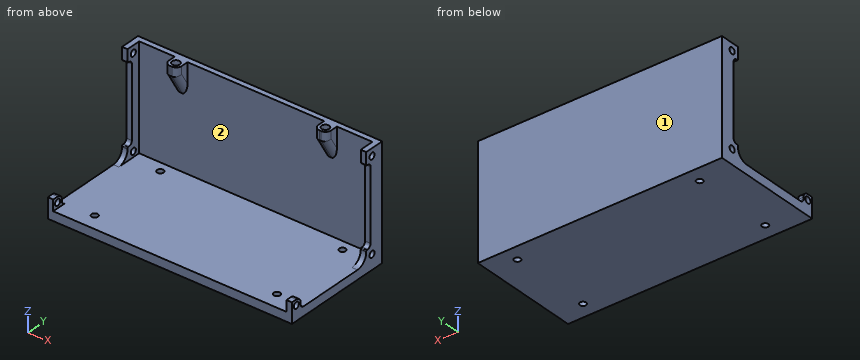
from build123d import *

# Parameters (mm, degrees)
SKETCH_W        = 134
SKETCH_H        = 62
PAD_DEPTH       = 5
SKETCH001_W     = 134
SKETCH001_H     = 3
PAD001_DEPTH    = 57
SKETCH002_W     = 7
SKETCH002_H     = 17
PAD002_DEPTH    = 7
POCKET_DEPTH    = 89
FILLET_R        = 3
SKETCH004_W     = 3
SKETCH004_H     = 57
PAD003_DEPTH    = 5
SKETCH005_W     = 3
SKETCH005_H     = 7
PAD004_DEPTH    = 3
SKETCH006_R     = 1.75
POCKET001_DEPTH = 134.001
SKETCH007_R     = 1.75
POCKET002_DEPTH = 5
SKETCH008_R     = 1.75
POCKET003_DEPTH = 5
SKETCH009_W     = 3
SKETCH009_H     = 6
PAD005_DEPTH    = 6
SKETCH010_R     = 1.75
POCKET004_DEPTH = 134.001
FILLET001_R     = 3
FILLET002_R     = 2
FILLET003_R     = 3
FILLET004_R     = 2
FILLET005_R     = 6
FILLET006_R     = 6
FILLET007_R     = 2
FILLET008_R     = 0.5
FILLET009_R     = 2
FILLET010_R     = 0.5
FILLET011_R     = 2
FILLET012_R     = 0.5
FILLET013_R     = 2
FILLET014_R     = 0.5
SKETCH011_R     = 1.75
POCKET005_DEPTH = 5
SKETCH012_R     = 2.1
POCKET006_DEPTH = 5


with BuildPart() as part:
    # Sketch → Pad (new body)
    with BuildSketch(Plane.XY):
        with Locations((67, -31)):
            Rectangle(SKETCH_W, SKETCH_H)
    extrude(amount=PAD_DEPTH)

    # Sketch001 (on Face6 of Pad) → Pad001 (join)
    with BuildSketch(Plane.XY.offset(5)):
        with Locations((67, -1.5)):
            Rectangle(SKETCH001_W, SKETCH001_H)
    extrude(amount=PAD001_DEPTH)

    # Sketch002 (on Face11 of Pad001) → Pad002 (join)
    with BuildSketch(Plane.XZ.offset(3)):
        with Locations((26, 53.5)):
            Rectangle(SKETCH002_W, SKETCH002_H)
        with Locations((108, 53.5)):
            Rectangle(SKETCH002_W, SKETCH002_H)
    extrude(amount=PAD002_DEPTH)

    # Sketch003 (on Face14 of Pad002) → Pocket (cut)
    with BuildSketch(Plane(origin=(22.5, 0, 0), x_dir=(0, -1, 0), z_dir=(-1, 0, 0))):
        Polygon((3, 45), (10, 57), (10, 45), align=None)
    extrude(amount=-POCKET_DEPTH, mode=Mode.SUBTRACT)

    # Fillet
    fillet_edges = [part.edges().sort_by_distance(p)[0] for p in [
        (104.5, -10, 59.5),
        (111.5, -10, 59.5),
        (111.5, -6.5, 51),
        (104.5, -6.5, 51),
        (22.5, -10, 59.5),
        (29.5, -10, 59.5),
        (29.5, -6.5, 51),
        (22.5, -6.5, 51),
    ]]
    fillet(fillet_edges, radius=FILLET_R)

    # Sketch004 (on Face1 of Fillet) → Pad003 (join)
    with BuildSketch(Plane.XZ.offset(3)):
        with Locations((1.5, 33.5)):
            Rectangle(SKETCH004_W, SKETCH004_H)
        with Locations((132.5, 33.5)):
            Rectangle(SKETCH004_W, SKETCH004_H)
    extrude(amount=PAD003_DEPTH)

    # Sketch005 (on Face32 of Pad003) → Pad004 (join)
    with BuildSketch(Plane.XZ.offset(8)):
        with Locations((1.5, 8.5)):
            Rectangle(SKETCH005_W, SKETCH005_H)
        with Locations((1.5, 58.5)):
            Rectangle(SKETCH005_W, SKETCH005_H)
        with Locations((132.5, 8.5)):
            Rectangle(SKETCH005_W, SKETCH005_H)
        with Locations((132.5, 58.5)):
            Rectangle(SKETCH005_W, SKETCH005_H)
    extrude(amount=PAD004_DEPTH)

    # Sketch006 (on Face44 of Pad004) → Pocket001 (cut, through all)
    with BuildSketch(Plane(origin=(0, 0, 0), x_dir=(0, -1, 0), z_dir=(-1, 0, 0))):
        with Locations((7, 8)):
            Circle(SKETCH006_R)
    extrude(amount=-POCKET001_DEPTH, mode=Mode.SUBTRACT)

    # Sketch007 (on Face46 of Pocket001) → Pocket002 (cut)
    with BuildSketch(Plane(origin=(0, 0, 0), x_dir=(0, -1, 0), z_dir=(-1, 0, 0))):
        with Locations((7, 58)):
            Circle(SKETCH007_R)
    extrude(amount=-POCKET002_DEPTH, mode=Mode.SUBTRACT)

    # Sketch008 (on Face45 of Pocket002) → Pocket003 (cut)
    with BuildSketch(Plane.YZ.offset(134)):
        with Locations((-7, 58)):
            Circle(SKETCH008_R)
    extrude(amount=-POCKET003_DEPTH, mode=Mode.SUBTRACT)

    # Sketch009 (on Face10 of Pocket003) → Pad005 (join)
    with BuildSketch(Plane.XY.offset(5)):
        with Locations((1.5, -59)):
            Rectangle(SKETCH009_W, SKETCH009_H)
        with Locations((132.5, -59)):
            Rectangle(SKETCH009_W, SKETCH009_H)
    extrude(amount=PAD005_DEPTH)

    # Sketch010 (on Face60 of Pad005) → Pocket004 (cut, through all)
    with BuildSketch(Plane.YZ.offset(134)):
        with Locations((-59, 8)):
            Circle(SKETCH010_R)
    extrude(amount=-POCKET004_DEPTH, mode=Mode.SUBTRACT)

    # Fillet001
    fillet001_edges = [part.edges().sort_by_distance(p)[0] for p in [
        (132.5, -56, 11),
    ]]
    fillet(fillet001_edges, radius=FILLET001_R)

    # Fillet002
    fillet002_edges = [part.edges().sort_by_distance(p)[0] for p in [
        (132.5, -56, 5),
    ]]
    fillet(fillet002_edges, radius=FILLET002_R)

    # Fillet003
    fillet003_edges = [part.edges().sort_by_distance(p)[0] for p in [
        (1.5, -56, 11),
    ]]
    fillet(fillet003_edges, radius=FILLET003_R)

    # Fillet004
    fillet004_edges = [part.edges().sort_by_distance(p)[0] for p in [
        (1.5, -56, 5),
    ]]
    fillet(fillet004_edges, radius=FILLET004_R)

    # Fillet005
    fillet005_edges = [part.edges().sort_by_distance(p)[0] for p in [
        (1.5, -11, 5),
    ]]
    fillet(fillet005_edges, radius=FILLET005_R)

    # Fillet006
    fillet006_edges = [part.edges().sort_by_distance(p)[0] for p in [
        (132.5, -11, 5),
    ]]
    fillet(fillet006_edges, radius=FILLET006_R)

    # Fillet007
    fillet007_edges = [part.edges().sort_by_distance(p)[0] for p in [
        (1.5, -8, 12),
    ]]
    fillet(fillet007_edges, radius=FILLET007_R)

    # Fillet008
    fillet008_edges = [part.edges().sort_by_distance(p)[0] for p in [
        (1.5, -11, 12),
    ]]
    fillet(fillet008_edges, radius=FILLET008_R)

    # Fillet009
    fillet009_edges = [part.edges().sort_by_distance(p)[0] for p in [
        (132.5, -8, 12),
    ]]
    fillet(fillet009_edges, radius=FILLET009_R)

    # Fillet010
    fillet010_edges = [part.edges().sort_by_distance(p)[0] for p in [
        (132.5, -11, 12),
    ]]
    fillet(fillet010_edges, radius=FILLET010_R)

    # Fillet011
    fillet011_edges = [part.edges().sort_by_distance(p)[0] for p in [
        (1.5, -8, 55),
    ]]
    fillet(fillet011_edges, radius=FILLET011_R)

    # Fillet012
    fillet012_edges = [part.edges().sort_by_distance(p)[0] for p in [
        (1.5, -11, 55),
    ]]
    fillet(fillet012_edges, radius=FILLET012_R)

    # Fillet013
    fillet013_edges = [part.edges().sort_by_distance(p)[0] for p in [
        (132.5, -8, 55),
    ]]
    fillet(fillet013_edges, radius=FILLET013_R)

    # Fillet014
    fillet014_edges = [part.edges().sort_by_distance(p)[0] for p in [
        (132.5, -11, 55),
    ]]
    fillet(fillet014_edges, radius=FILLET014_R)

    # Sketch011 (on Face13 of Fillet014) → Pocket005 (cut)
    with BuildSketch(Plane.XY.offset(5)):
        with Locations((19, -8.5)):
            Circle(SKETCH011_R)
        with Locations((19, -53.5)):
            Circle(SKETCH011_R)
        with Locations((119, -53.5)):
            Circle(SKETCH011_R)
        with Locations((119, -8.5)):
            Circle(SKETCH011_R)
    extrude(amount=-POCKET005_DEPTH, mode=Mode.SUBTRACT)

    # Sketch012 (on Face73 of Pocket005) → Pocket006 (cut)
    with BuildSketch(Plane.XY.offset(62)):
        with Locations((26, -6.5)):
            Circle(SKETCH012_R)
        with Locations((108, -6.5)):
            Circle(SKETCH012_R)
    extrude(amount=-POCKET006_DEPTH, mode=Mode.SUBTRACT)


solid = part.part
Work out the finished part from the listing and answer in its coordinate system (mm). Face numbers are marked on the shaded views. Give positions to 0.01 mm unless a question says otherwise; leave off trailing zeros. Order: outer loops, then holes, each group sorted by start corner. A loop starts at its lowest first (then second) coordinate and runs counter-clockwise, first axis right, second up. Notation, with made-up numbers: M -16.75,-14.5 L -1.75,-14.5 A9 cw -1.75,-7.5 Z; hole C -12,-4.75 d1. An arc over 180 degrees is marked long. Return JSON: item names as keys, results as strings.
Q1. The mould has two halves that part along X. Classify the marked faces 1 and 2: pulls with the +X half, pulls with the -X half, needs draft (parallel to the pull), parting line crosses it, or undercut.
Answer below:
{"face 1": "needs draft", "face 2": "undercut"}
Q2. Each of these flat-tipped pins is pushed along its axis until it touches: pin 1 (0.5 mm diameter, centred on x = 108, z = 59, fed in from -Y); pin 2 (10 mm diameter, centred on x = 89, y = -42, fed in from -Z); pin 3 (0.9 mm diameter, centred on x = 132, z = 40.5, fed in from -Y); pin 4 (2.5 mm diameter, centred on x = 1.5, y = -61, fed in from +Z). Where does it stop, or does it pass through?
Answer below:
{"pin 1": "stops at y = -10", "pin 2": "stops at z = 0", "pin 3": "stops at y = -8", "pin 4": "stops at z = 11"}
Q3. Find section B-B, the plane x = 50.5. Write down the section's boundary in (y, z), and give its area (3 significant figures).
Answer below:
{"outline": "M -62,0 L 0,0 L 0,62 L -3,62 L -3,5 L -62,5 Z", "area": "481 mm^2"}
Q4. Find the intervals of material crossed by line 1 along Y through (x, z) = (19, 3.55); line 2 along Z through (x, y) = (0.7, -7); line 3 along Z through (x, y) = (132.6, -59), in increasing order. Write a range as [from, to].
Answer below:
{"line 1": "y = [-62, -55.25], [-51.75, -10.25], [-6.75, 0]", "line 2": "z = [0, 6.25], [9.75, 56.25], [59.75, 62]", "line 3": "z = [0, 6.25], [9.75, 11]"}
Q5. Find section C-C, the plane y = -50. Write down the section's boundary in (x, z).
Answer below:
{"outline": "M 0,0 L 134,0 L 134,5 L 0,5 Z"}
Q6. Find section A-A, the plane z = 36. Write down the section's boundary in (x, y).
Answer below:
{"outline": "M 0,-8 L 3,-8 L 3,-3 L 131,-3 L 131,-8 L 134,-8 L 134,0 L 0,0 Z"}
